Check sheet for the drawn part. Datum: minimum x, y, z corner. Units: mm. A direction names the side the tool comes from. Give positions to 0.01 mm unless a question says otherwise; leave off trailing zeros. Loops run counter-clockwise (first coordinate to the right, second up) from the corner with the lowest first, then second, coordinate; pieces in that order, holes last. Notation, with made-up numbers: (53.25, -31) -> (96.25, -31) arc R21 cw to (96.25, 8) -> close; hole circle Ø6 at (31.25, 84). An arc over 180 degrees is marked (long way). One line per question, with ' | ' between items.
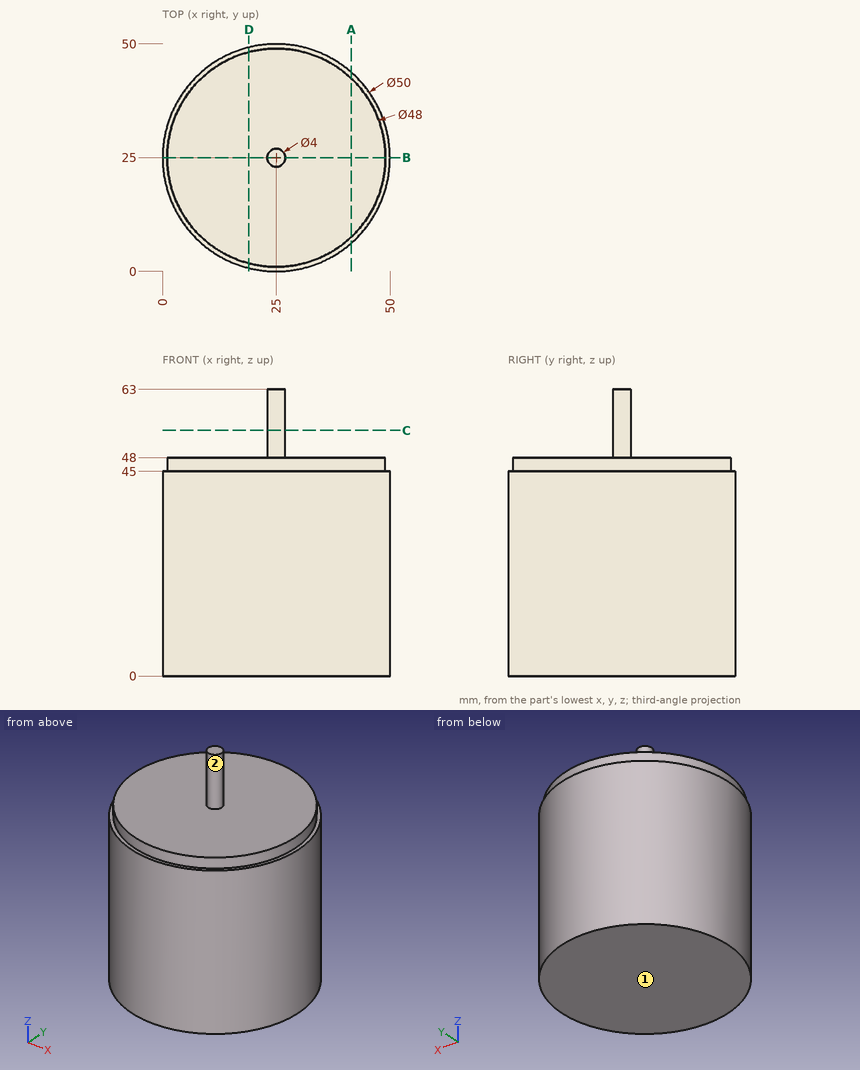
Item 1: Depth check by flat-ended pin: pin 1 Ø10 at (x, z) = (36.5, 21) entering from -Y; pin 2 Ø5 at (x, y) = (33, 42.5) entering from +Z; pin 3 Ø6 at (x, z) = (13, 20.5) entering from -Y. Enter the tip coordinate at first touch or a pass-through.
Result:
pin 1: y = 0.86 | pin 2: z = 48 | pin 3: y = 1.68
Item 2: Sectioned sample at A-A (x = 41.5). Record the cut outline in (y, z).
Result:
outline: (6.22, 0) -> (43.78, 0) -> (43.78, 45) -> (42.43, 45) -> (42.43, 48) -> (7.57, 48) -> (7.57, 45) -> (6.22, 45) -> close
Item 3: Scan lines: probe 1 along Z at (x, y) = (44.5, 35); probe 2 along X at (y, z) = (39, 18.5); probe 3 along Y at (x, z) = (11.5, 24). Record each from-to range of solid material in increasing order.
Result:
probe 1: 0 to 48 | probe 2: 4.29 to 45.71 | probe 3: 3.96 to 46.04
Item 4: Sectioned sample at D-D (x = 19). Record the cut outline in (y, z).
Result:
outline: (0.73, 0) -> (49.27, 0) -> (49.27, 45) -> (48.24, 45) -> (48.24, 48) -> (1.76, 48) -> (1.76, 45) -> (0.73, 45) -> close
Item 5: Set-up check for the marked faces 1 and 2: record each of +Z, -Z, +X, -X, +Y, -Y from which the full face is reachable in a straight line by a thin tool's end or side.
Result:
face 1: -Z, +X, -X, +Y, -Y | face 2: +Z
Item 6: Sectioned sample at B-B (y = 25). Record the cut outline in (x, z).
Result:
outline: (0, 0) -> (50, 0) -> (50, 45) -> (49, 45) -> (49, 48) -> (27, 48) -> (27, 63) -> (23, 63) -> (23, 48) -> (1, 48) -> (1, 45) -> (0, 45) -> close
Item 7: Sectioned sample at C-C (z = 54). Record the cut outline in (x, y), plus the area to 3 significant figures.
Result:
outline: circle Ø4 at (25, 25) | area: 12.6 mm2
